Check sheet for the modelled part. Datum: model origin and axes. Units: mm. A direction names the side the tool comes from. Coordinates: 2 decimals unless noted, no trailing zeros. Loops run counter-clockwise (first coordinate to the right, second up) from the corner with the lowest first, then second, coordinate; pieces in that order, holes last. Notation, with made-up numbers: (-30, 37.25) -> (-10, 37.25) arc R19 ccw to (-10, 69.25) -> close; hole circle Ø10 at (5, -11). An arc over 180 degrees is marked (long way). Use CSV: the item, a comma, the result in double quotes.
```python
from build123d import *

# Parameters (mm, degrees)
SKETCH1_R           = 3.5
BOSS_EXTRUDE1_DEPTH = 1
DOME1_FACE_RADIUS   = 3.5
DOME1_HEIGHT        = 0.75
SKETCH2_R           = 1.25
BOSS_EXTRUDE2_DEPTH = 8


with BuildPart() as part:
    # Sketch1 → Boss-Extrude1 (new body)
    with BuildSketch(Plane(origin=(0, 0, 0), x_dir=(1, 0, 0), z_dir=(0, 1, 0))):
        with Locations(Location((0, 0, 0), (0, 0, 270))):
            Circle(SKETCH1_R)
    extrude(amount=BOSS_EXTRUDE1_DEPTH)

    # Dome1: a dome of height H over a round flat face of radius A is a cap of a sphere of radius (A * A + H * H) / (2 * H)
    dome1_r = (DOME1_FACE_RADIUS * DOME1_FACE_RADIUS + DOME1_HEIGHT * DOME1_HEIGHT) / (2 * DOME1_HEIGHT)
    dome1_base = Plane((0, 1, 0), z_dir=(0, 1, 0))
    with Locations(dome1_base.offset(DOME1_HEIGHT - dome1_r)):
        dome1_ball = Sphere(dome1_r, mode=Mode.PRIVATE)
    add(split(dome1_ball, bisect_by=dome1_base, keep=Keep.TOP, mode=Mode.PRIVATE))

    # Sketch2 → Boss-Extrude2 (add)
    with BuildSketch(Plane.XZ):
        with Locations(Location((0, 0, 0), (0, 0, 90))):
            Circle(SKETCH2_R)
    extrude(amount=BOSS_EXTRUDE2_DEPTH)


solid = part.part
```
1) Cross-section at D-D on x = 2.25. Record the boundary of the cut face in (y, z), and give its area (3 significant figures).
Answer below:
outline,"(0, -2.68) -> (1, -2.68) arc R8.24 ccw to (1, 2.68) -> (0, 2.68) -> close"
area,"6.97 mm²"
2) Cross-section at A-A on x = 0. Record the boundary of the cut face in (y, z), and give its area (3 significant figures).
Answer below:
outline,"(-8, -1.25) -> (0, -1.25) -> (0, -3.5) -> (1, -3.5) arc R8.54 ccw to (1, 3.5) -> (0, 3.5) -> (0, 1.25) -> (-8, 1.25) -> close"
area,"30.5 mm²"
3) Thickness scan on line 1 along X through (y, z) = (-4, 0); line 2 along Y through (x, z) = (1, -2.25); line 3 along Y through (x, z) = (-2.25, -2). Record the ranges inside material, lowest first. Write a range as from..to.
Answer below:
line 1,"x = -1.25..1.25"
line 2,"y = 0..1.39"
line 3,"y = 0..1.2"
4) Go/stop test with flat-tipped pins: pin 1 Ø4 at (x, y) = (-2, -4.5) entering from -Z; pin 2 Ø1 at (x, z) = (-1, -1.5) entering from +Y. Record where each tip stops, or that it passes through.
Answer below:
pin 1,"stops at z = -1.25"
pin 2,"stops at y = 1.65"
5) Cross-section at C-C on y = -3.25. Record the boundary of the cut face in (x, z), and give its area (3 significant figures).
Answer below:
outline,"circle Ø2.5 at (0, 0)"
area,"4.91 mm²"
6) Access from +Z, -Z, +X, -X, +Y, -Y to the whole of each face (thin tool, end or side, straight path). Record for faces 1 (the flat face through (0, -8, 0)), 2 (the cylindrical face through (1.22, -3.94, -0.27)).
Answer below:
face 1,"+Z, -Z, +X, -X, -Y"
face 2,"-Y"
7) Cross-section at B-B on z = 0. Record the boundary of the cut face in (x, y), and give its area (3 significant figures).
Answer below:
outline,"(-3.5, 0) -> (-1.25, 0) -> (-1.25, -8) -> (1.25, -8) -> (1.25, 0) -> (3.5, 0) -> (3.5, 1) arc R8.54 ccw to (-3.5, 1) -> close"
area,"30.5 mm²"
